Study the drawing (mm; zero at the part's minimum x, y, z) and answer. Round coordinates to 2 decimals unless told otherwise and drop trailing zeros. Write each loop counter-clockwise with the first axis right and the second up, starting at its lowest first coordinate (ties: lowest second). Pieces come first, ordered by that corner, then holes.
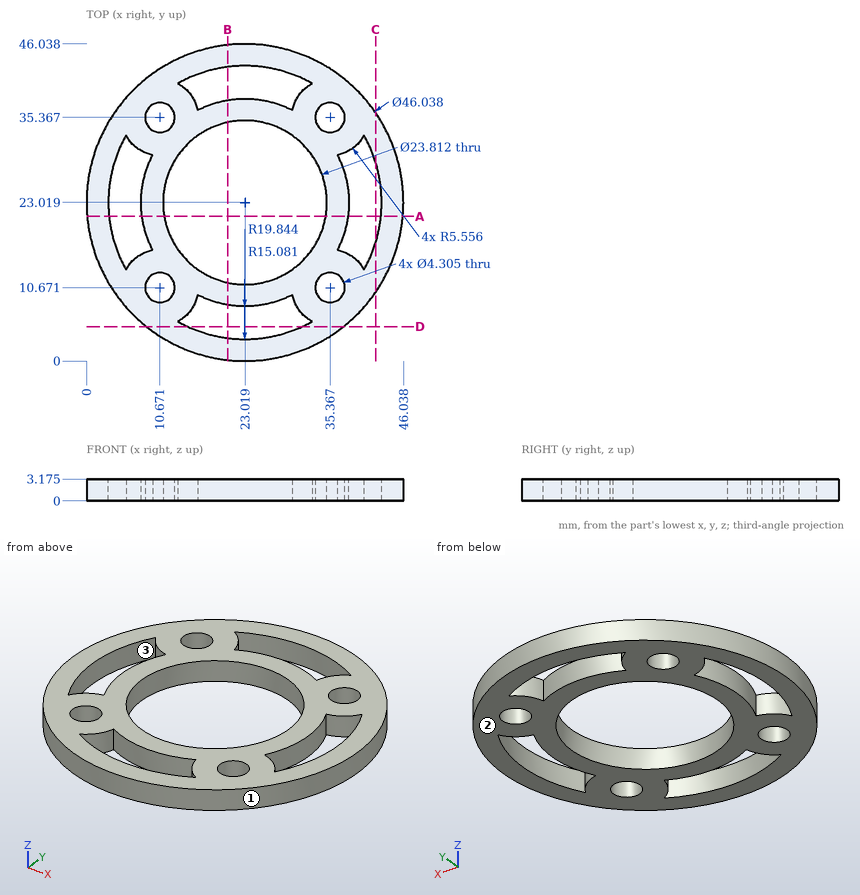
Q1. Given pin 1 (10 mm diameter, centred on x = 18, y = 19.5, fed in from +Z), flat-ended and moving along its own axis, determine where the tip first touches the part or whether it passes through.
Q2. Find section A-A (y = 21). Determine the outline of the cut face in (x, z) (1 decimal).
Q3. The mould has two halves that part along Y. Classify the marked faces 1, 2 and 3: +Y half, -Y half, draft (parallel to the pull), parting line (faces both ways), or undercut.
Q4. Find the intervals of material crossed by L1, parallel to X at y = 18, z = 2.75 (1 decimal); L2, parallel to Y at x = 25, z = 1.85 (1 decimal); L3, parallel to X at y = 17, z = 1.3 (1 decimal), in increasing order.
Q5. Find section B-B (x = 20.5). Count the separate pieces of the cut face and the enclosed holes in it.
Q6. Find section C-C (x = 42). Determine the outline of the cut face in (y, z) (1 decimal).
Q7. Find section D-D (y = 5). Determine the outline of the cut face in (x, z) (1 decimal).
Report:
1. pin 1: passes through
2. outline: (0.1, 0) - (3.3, 0) - (3.3, 3.2) - (0.1, 3.2) - close; (8.1, 0) - (11.3, 0) - (11.3, 3.2) - (8.1, 3.2) - close; (34.8, 0) - (38, 0) - (38, 3.2) - (34.8, 3.2) - close; (42.8, 0) - (45.9, 0) - (45.9, 3.2) - (42.8, 3.2) - close
3. face 1: parting line
3. face 2: draft
3. face 3: undercut
4. L1: x = 0.6 to 3.8, 8.8 to 12.2, 33.8 to 37.2, 42.2 to 45.5
4. L2: y = 0.1 to 3.3, 8.1 to 11.3, 34.8 to 38, 42.8 to 46
4. L3: x = 0.8 to 4.1, 9.2 to 12.7, 33.3 to 36.8, 41.9 to 45.2
5. separate pieces: 4
5. enclosed holes: 0
6. outline: (10, 0) - (17.2, 0) - (17.2, 3.2) - (10, 3.2) - close; (28.8, 0) - (36, 0) - (36, 3.2) - (28.8, 3.2) - close
7. outline: (8.7, 0) - (14.7, 0) - (14.7, 3.2) - (8.7, 3.2) - close; (31.3, 0) - (37.3, 0) - (37.3, 3.2) - (31.3, 3.2) - close
